The model under review builds one solid part; all positions refer to its coordinate system, in mm. Coordinates: 2 decimals unless noted, no trailing zeros. Write each loop counter-clockwise with the first axis right and the second up, starting at its lowest first coordinate (ties: lowest second). Pieces come first, ordered by that corner, then holes. Notation, with made-up numbers: M -39.5,60 L -9.5,60 A11 ccw -9.5,69 Z; hole C 22,40 d1. An arc over 180 degrees is marked long. Answer as a JSON object with one key per item and string values.
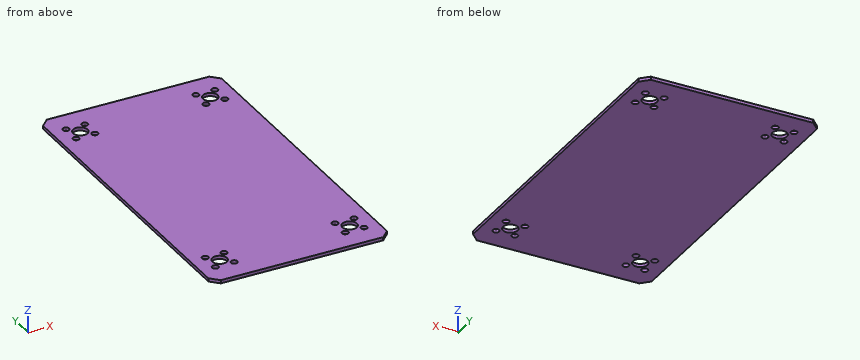
```python
from build123d import *

# Parameters (mm, degrees)
SKETCH1_W           = 110
SKETCH1_H           = 200
BOSS_EXTRUDE1_DEPTH = 2
SKETCH6_R           = 4.5
SKETCH6_R_2         = 1.95
LEANDUT_HOLES_DEPTH = 115.144645078
CHAMFER1_SIZE       = 5


with BuildPart() as part:
    # Sketch1 → Boss-Extrude1 (new body)
    with BuildSketch(Plane.XY):
        Rectangle(SKETCH1_W, SKETCH1_H)
    extrude(amount=BOSS_EXTRUDE1_DEPTH)

    # Sketch6 → Leandut_holes (cut, through all)
    with BuildSketch(Plane.XY.offset(2)):
        with Locations((-40, 80)):
            Circle(SKETCH6_R)
        with Locations((-45.8, 85.8)):
            Circle(SKETCH6_R_2)
        with Locations(Location((-45.8, 74.2, 0), (0, 0, 180))):
            Circle(SKETCH6_R_2)
        with Locations((-34.2, 74.2)):
            Circle(SKETCH6_R_2)
        with Locations(Location((-34.2, 85.8, 0), (0, 0, 180))):
            Circle(SKETCH6_R_2)
        with Locations((34.2, 85.8)):
            Circle(SKETCH6_R_2)
        with Locations(Location((34.2, 74.2, 0), (0, 0, 180))):
            Circle(SKETCH6_R_2)
        with Locations((45.8, 74.2)):
            Circle(SKETCH6_R_2)
        with Locations(Location((45.8, 85.8, 0), (0, 0, 180))):
            Circle(SKETCH6_R_2)
        with Locations(Location((40, 80, 0), (0, 0, 180))):
            Circle(SKETCH6_R)
        with Locations((40, -80)):
            Circle(SKETCH6_R)
        with Locations((45.8, -85.8)):
            Circle(SKETCH6_R_2)
        with Locations(Location((45.8, -74.2, 0), (0, 0, 180))):
            Circle(SKETCH6_R_2)
        with Locations((34.2, -74.2)):
            Circle(SKETCH6_R_2)
        with Locations(Location((34.2, -85.8, 0), (0, 0, 180))):
            Circle(SKETCH6_R_2)
        with Locations((-34.2, -85.8)):
            Circle(SKETCH6_R_2)
        with Locations(Location((-34.2, -74.2, 0), (0, 0, 180))):
            Circle(SKETCH6_R_2)
        with Locations((-45.8, -74.2)):
            Circle(SKETCH6_R_2)
        with Locations(Location((-45.8, -85.8, 0), (0, 0, 180))):
            Circle(SKETCH6_R_2)
        with Locations(Location((-40, -80, 0), (0, 0, 180))):
            Circle(SKETCH6_R)
    extrude(amount=-LEANDUT_HOLES_DEPTH, mode=Mode.SUBTRACT)

    # Chamfer1
    chamfer1_edges = [part.edges().sort_by_distance(p)[0] for p in [
        (55, -100, 1),
        (-55, -100, 1),
        (-55, 100, 1),
        (55, 100, 1),
    ]]
    chamfer(chamfer1_edges, length=CHAMFER1_SIZE)


solid = part.part
```
(1) Add section C-C on z = 1.4. Count the separate pieces of the cut face and the enclosed holes in it, and give its area (3 significant figures).
Results list:
{"separate pieces": "1", "enclosed holes": "20", "area": "21,500 mm²"}
(2) Add section B-B on y = -80. Give the boundary of the cut face in (x, z), and give its area (3 significant figures).
Results list:
{"outline": "M -55,0 L -44.5,0 L -44.5,2 L -55,2 Z; M -35.5,0 L 35.5,0 L 35.5,2 L -35.5,2 Z; M 44.5,0 L 55,0 L 55,2 L 44.5,2 Z", "area": "184 mm²"}
(3) For pin 1 Ø10.5 at (x, y) = (40, -80) entering from -Z, flat-tipped, find the tip position at first contact; note if it passes through.
Results list:
{"pin 1": "z = 0"}
(4) Add section A-A on x = 40. Give the boundary of the cut face in (y, z).
Results list:
{"outline": "M -100,0 L -84.5,0 L -84.5,2 L -100,2 Z; M -75.5,0 L 75.5,0 L 75.5,2 L -75.5,2 Z; M 84.5,0 L 100,0 L 100,2 L 84.5,2 Z"}
(5) Wall thickness on line 1 along Y through (x, z) = (34.2, 0.55); line 2 along Y through (x, z) = (-40, 1.45); line 3 along X through (y, z) = (79.5, 1.3): over which ranges is each line inside the solid? List them lowest first. Write a range as from..to.
Results list:
{"line 1": "-100..-87.75, -83.85..-76.15, -72.25..72.25, 76.15..83.85, 87.75..100", "line 2": "-100..-84.5, -75.5..75.5, 84.5..100", "line 3": "-55..-44.47, -35.53..35.53, 44.47..55"}
